```python
from build123d import *

# Parameters (mm, degrees)
SKETCH_1_R      = 25
EXTRUDE_1_DEPTH = 5
SKETCH_3_R      = 22.5
SKETCH_3_R_2    = 1.524
SKETCH_3_R_3    = 1.7272
SKETCH_3_R_4    = 5.08
EXTRUDE_2_DEPTH = 2


with BuildPart() as part:
    # 草圖1 → 填料-伸長1 (new body)
    with BuildSketch(Plane(origin=(0, 0, 0), x_dir=(1, 0, 0), z_dir=(0, 1, 0))):
        with Locations(Location((0, 0, 0), (0, 0, 270))):
            Circle(SKETCH_1_R)
        with BuildLine():
            Line((-19.962936653, -2.035103236), (-19.935577611, -2.287625478))
            ThreePointArc((-19.935577611, -2.287625478), (-18.582614267, -4.760555699), (-15.877298983, -5.552491873))
            Line((-15.877298983, -5.552491873), (-7.039020507, -4.594925386))
            ThreePointArc((-7.039020507, -4.594925386), (-4.333705223, -5.38686156), (-2.980741879, -7.859791782))
            Line((-2.980741879, -7.859791782), (-2.023175392, -16.698070258))
            ThreePointArc((-2.023175392, -16.698070258), (-0.670212048, -19.171000479), (2.035103236, -19.962936653))
            Line((2.035103236, -19.962936653), (2.287625478, -19.935577611))
            ThreePointArc((2.287625478, -19.935577611), (4.760555699, -18.582614267), (5.552491873, -15.877298983))
            Line((5.552491873, -15.877298983), (4.594925386, -7.039020507))
            ThreePointArc((4.594925386, -7.039020507), (5.38686156, -4.333705223), (7.859791782, -2.980741879))
            Line((7.859791782, -2.980741879), (16.698070258, -2.023175392))
            ThreePointArc((16.698070258, -2.023175392), (19.171000479, -0.670212048), (19.962936653, 2.035103236))
            Line((19.962936653, 2.035103236), (19.935577611, 2.287625478))
            ThreePointArc((19.935577611, 2.287625478), (18.582614267, 4.760555699), (15.877298983, 5.552491873))
            Line((15.877298983, 5.552491873), (7.039020507, 4.594925386))
            ThreePointArc((7.039020507, 4.594925386), (4.333705223, 5.38686156), (2.980741879, 7.859791782))
            Line((2.980741879, 7.859791782), (2.023175392, 16.698070258))
            ThreePointArc((2.023175392, 16.698070258), (0.670212048, 19.171000479), (-2.035103236, 19.962936653))
            Line((-2.035103236, 19.962936653), (-2.287625478, 19.935577611))
            ThreePointArc((-2.287625478, 19.935577611), (-4.760555699, 18.582614267), (-5.552491873, 15.877298983))
            Line((-5.552491873, 15.877298983), (-4.594925386, 7.039020507))
            ThreePointArc((-4.594925386, 7.039020507), (-5.38686156, 4.333705223), (-7.859791782, 2.980741879))
            Line((-7.859791782, 2.980741879), (-16.698070258, 2.023175392))
            ThreePointArc((-16.698070258, 2.023175392), (-19.171000479, 0.670212048), (-19.962936653, -2.035103236))
        make_face(mode=Mode.SUBTRACT)
    extrude(amount=EXTRUDE_1_DEPTH)

    # 草圖3 → 填料-伸長2 (add)
    with BuildSketch(Plane(origin=(0, 0, 0), x_dir=(1, 0, 0), z_dir=(0, 1, 0))):
        Circle(SKETCH_3_R)
        with Locations(Location((16.982120786, 1.839895607, 0), (0, 0, 270))):
            Circle(SKETCH_3_R_2, mode=Mode.SUBTRACT)
        with Locations(Location((9.217061839, 0.998605051, 0), (0, 0, 270))):
            Circle(SKETCH_3_R_3, mode=Mode.SUBTRACT)
        with Locations(Location((1.839895607, -16.982120786, 0), (0, 0, 270))):
            Circle(SKETCH_3_R_2, mode=Mode.SUBTRACT)
        with Locations(Location((0.861809838, -7.954450629, 0), (0, 0, 270))):
            Circle(SKETCH_3_R_3, mode=Mode.SUBTRACT)
        with Locations(Location((0, 0, 0), (0, 0, 270))):
            Circle(SKETCH_3_R_4, mode=Mode.SUBTRACT)
        with Locations(Location((-16.982120786, -1.839895607, 0), (0, 0, 270))):
            Circle(SKETCH_3_R_2, mode=Mode.SUBTRACT)
        with Locations(Location((-9.217061839, -0.998605051, 0), (0, 0, 270))):
            Circle(SKETCH_3_R_3, mode=Mode.SUBTRACT)
        with Locations(Location((-1.839895607, 16.982120786, 0), (0, 0, 270))):
            Circle(SKETCH_3_R_2, mode=Mode.SUBTRACT)
        with Locations(Location((-0.861809838, 7.954450629, 0), (0, 0, 270))):
            Circle(SKETCH_3_R_3, mode=Mode.SUBTRACT)
    extrude(amount=EXTRUDE_2_DEPTH)


solid = part.part
```
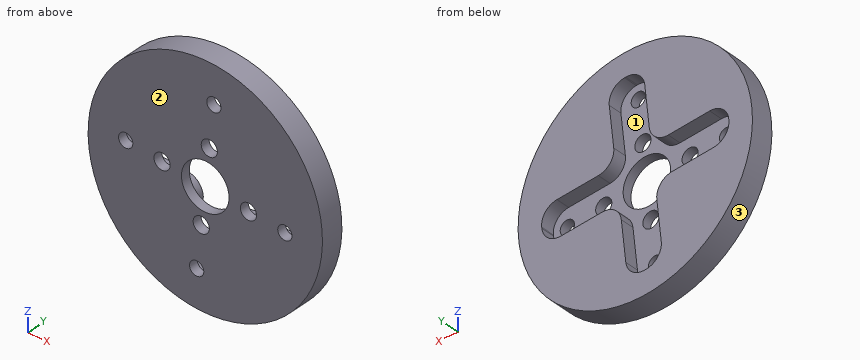
Can you work these out from the model? Positions are in its coordinate system, mm. Face numbers are marked on the shaded views. Give positions to 0.01 mm unless a question says otherwise; leave off trailing zeros. Order: outer loops, then holes, each group sorted by start corner. A loop starts at its lowest first (then second) coordinate and runs counter-clockwise, first axis right, second up. Notation, with made-up numbers: (67.25, 40.5) - (121.25, 40.5) arc R31 cw to (121.25, 69.5) - close; hole circle Ø11 at (85.5, -27). An arc over 180 degrees is marked (long way). Use a Markdown table: item, result. Add a question column.
Q1. If we section it at A-A on y = 4.1: Write out the boundary of the cut face in (x, z).
Q2. If we section it at D-D on x = 12.5: Write out the boundary of the cut face in (y, z), plus the area to 3 significant figures.
Q3. If we section it at B-B on z = -10.5: Write out the boundary of the cut face in (x, y).
Q4. I'm going to push flat-ended pins straight in: pin 1 (5.5 mm diameter, centred on x = 0.86, z = 7.95, fed in from -Y); pin 2 (1.5 mm diameter, centred on y = 3.5, z = -14.5, fed in from +X); pin 3 (6 mm diameter, centred on x = 0, z = 0, fed in from -Y); pin 4 (5 mm diameter, centred on x = -16.98, z = 1.84, fed in from +Y). Where does each tip first touch, or does it pass through?
Q5. If we section it at C-C on y = 0.8: Count the separate pieces of the cut face and the enclosed holes in it, plus the area to 3 significant figures.
Q6. If we mould it in two halves opening along Z, with no side actions, what happens to the marked faces 1, 2 and 3? For each: released by +Z, released by -Z, zero draft, split by the parting line, or undercut.
Q7. Please list where these lines run through material, in increasing order: line 1 along X through (y, z) = (1.8, -3); line 2 along X through (y, z) = (3.25, -8.5); line 3 along X through (y, z) = (2.7, -15.5).
Answers follow:
| question | item | result |
|---|---|---|
| 1 | outline | circle Ø50 at (0, 0); hole (-19.96, 2.04) arc R3.68 ccw to (-16.7, -2.02) - (-7.86, -2.98) arc R3.68 cw to (-4.59, -7.04) - (-5.55, -15.88) arc R3.68 ccw to (-2.29, -19.94) - (-2.04, -19.96) arc R3.68 ccw to (2.02, -16.7) - (2.98, -7.86) arc R3.68 cw to (7.04, -4.59) - (15.88, -5.55) arc R3.68 ccw to (19.94, -2.29) - (19.96, -2.04) arc R3.68 ccw to (16.7, 2.02) - (7.86, 2.98) arc R3.68 cw to (4.59, 7.04) - (5.55, 15.88) arc R3.68 ccw to (2.29, 19.94) - (2.04, 19.96) arc R3.68 ccw to (-2.02, 16.7) - (-2.98, 7.86) arc R3.68 cw to (-7.04, 4.59) - (-15.88, 5.55) arc R3.68 ccw to (-19.94, 2.29) - close |
| 2 | outline | (0, -21.65) - (5, -21.65) - (5, -5.19) - (2, -5.19) - (2, 2.48) - (5, 2.48) - (5, 21.65) - (0, 21.65) - close |
| 2 | area | 194 mm^2 |
| 3 | outline | (-22.69, 0) - (22.69, 0) - (22.69, 5) - (2.69, 5) - (2.69, 2) - (-4.97, 2) - (-4.97, 5) - (-22.69, 5) - close |
| 4 | pin 1 | stops at y = 0 |
| 4 | pin 2 | stops at x = 20.88 |
| 4 | pin 3 | passes through |
| 4 | pin 4 | stops at y = 2 |
| 5 | separate pieces | 1 |
| 5 | enclosed holes | 9 |
| 5 | area | 1,820 mm^2 |
| 6 | face 1 | undercut |
| 6 | face 2 | zero draft |
| 6 | face 3 | split by the parting line |
| 7 | line 1 | x = -24.82 to -4.1, 4.1 to 15.99, 17.97 to 24.82 |
| 7 | line 2 | x = -23.51 to -4.75, 2.91 to 23.51 |
| 7 | line 3 | x = -19.62 to -5.51, 2.15 to 19.62 |
